Build history of the part. All positions in model axes, mm. A direction names the side the tool comes from. Give positions to 0.01 mm unless a question says otherwise; leave off trailing zeros. Order: outer loops, then holes, each group sorted by start corner. A loop starts at its lowest first (then second) coordinate and runs counter-clockwise, first axis right, second up. Notation, with made-up numbers: (-10, 52.25) - (45, 52.25) arc R22 cw to (45, 58.25) - close; hole circle Ø2 at (86, 55). An arc over 180 degrees is marked (long way). Use a Markdown table: item, result.
from build123d import *

# Parameters (mm, degrees)
F1_DEPTH       = 3
F2_D           = 8
F2_CSINK_D     = 16
F2_CSINK_ANGLE = 90


with BuildPart() as f1:
    # F0 (on Front) → F1 (new body)
    with BuildSketch(Plane.XZ):
        with BuildLine():
            ThreePointArc((-42.428788, 22.197763), (-22.393428, 40.636528), (0.736568, 26.269656))
            Line((0.736568, 26.269656), (7.82161, 7.734496))
            Line((7.82161, 7.734496), (445.831745, 440.866256))
            Line((445.831745, 440.866256), (409.571118, 551.809463))
            ThreePointArc((409.571118, 551.809463), (403.393924, 553.012383), (397.791506, 555.879027))
            Line((397.791506, 555.879027), (-153.711431, 555.879027))
            Line((-153.711431, 555.879027), (-163.711431, 555.879027))
            Line((-163.711431, 555.879027), (-176.433934, 530.299822))
            Line((-176.433934, 530.299822), (-292.672837, 296.595913))
            Line((-292.672837, 296.595913), (-429.805557, 108.635613))
            ThreePointArc((-429.805557, 108.635613), (-433.055197, 105.145969), (-437.038546, 102.524765))
            Line((-437.038546, 102.524765), (-467.979575, 87.098137))
            ThreePointArc((-467.979575, 87.098137), (-479.031049, 77.063624), (-483.216559, 62.73505))
            Line((-483.216559, 62.73505), (-444.218322, 62.364245))
            ThreePointArc((-444.218322, 62.364245), (-439.992581, 60.566627), (-438.27564, 56.307469))
            ThreePointArc((-438.27564, 56.307469), (-440.073258, 52.081729), (-444.332415, 50.364787))
            Line((-444.332415, 50.364787), (-483.330653, 50.735592))
            Line((-483.330653, 50.735592), (-473.742625, 39.200006))
            ThreePointArc((-473.742625, 39.200006), (-462.016917, 29.862605), (-447.542263, 25.968544))
            Line((-447.542263, 25.968544), (-119.640526, 6.942116))
            ThreePointArc((-119.640526, 6.942116), (-119.539343, 30.38703), (-113.982147, 53.164032))
            ThreePointArc((-113.982147, 53.164032), (-112.028876, 55.605369), (-109.00742, 56.409233))
            Line((-109.00742, 56.409233), (-91.138541, 55.372396))
            ThreePointArc((-91.138541, 55.372396), (-94.609764, 47.818656), (-97.278364, 39.945477))
            ThreePointArc((-97.278364, 39.945477), (-100.140537, 22.963258), (-99.30184, 5.761968))
            Line((-99.30184, 5.761968), (-45.922757, 2.664658))
            Line((-45.922757, 2.664658), (-42.428788, 22.197763))
        make_face()
        with BuildLine():
            ThreePointArc((-219.185589, 82.205842), (-234.185589, 97.205842), (-219.185589, 112.205842))
            Line((-219.185589, 112.205842), (-139.185589, 112.205842))
            ThreePointArc((-139.185589, 112.205842), (-124.185589, 97.205842), (-139.185589, 82.205842))
            Line((-139.185589, 82.205842), (-219.185589, 82.205842))
        make_face(mode=Mode.SUBTRACT)
        with BuildLine():
            ThreePointArc((-238.884885, 257.620199), (-269.539195, 249.087128), (-278.072266, 279.741438))
            Line((-278.072266, 279.741438), (-223.998126, 375.532812))
            ThreePointArc((-223.998126, 375.532812), (-193.343817, 384.065883), (-184.810746, 353.411573))
            Line((-184.810746, 353.411573), (-238.884885, 257.620199))
        make_face(mode=Mode.SUBTRACT)
        with BuildLine():
            ThreePointArc((-109.00742, 56.409233), (-99.197738, 50.987949), (-97.278364, 39.945477))
            ThreePointArc((-97.278364, 39.945477), (-94.609764, 47.818656), (-91.138541, 55.372396))
            Line((-91.138541, 55.372396), (-109.00742, 56.409233))
        make_face()
        with BuildLine():
            Line((-153.711431, 555.879027), (397.791506, 555.879027))
            ThreePointArc((397.791506, 555.879027), (388.241023, 574.279027), (397.791506, 592.679027))
            Line((397.791506, 592.679027), (-153.711431, 592.679027))
            ThreePointArc((-153.711431, 592.679027), (-135.311431, 574.279027), (-153.711431, 555.879027))
        make_face()
        with BuildLine():
            Line((-153.711431, 592.679027), (397.791506, 592.679027))
            ThreePointArc((397.791506, 592.679027), (403.393924, 595.545671), (409.571118, 596.748591))
            Line((409.571118, 596.748591), (418.046209, 622.679027))
            Line((418.046209, 622.679027), (406.046209, 622.679027))
            ThreePointArc((406.046209, 622.679027), (403.924889, 623.557707), (403.046209, 625.679027))
            ThreePointArc((403.046209, 625.679027), (403.924889, 627.800347), (406.046209, 628.679027))
            Line((406.046209, 628.679027), (420.007247, 628.679027))
            Line((420.007247, 628.679027), (445.831745, 707.691799))
            Line((445.831745, 707.691799), (7.82161, 1140.823559))
            Line((7.82161, 1140.823559), (0.736568, 1122.288398))
            ThreePointArc((0.736568, 1122.288398), (-22.393428, 1107.921526), (-42.428788, 1126.360291))
            Line((-42.428788, 1126.360291), (-45.922757, 1145.893396))
            Line((-45.922757, 1145.893396), (-447.542263, 1122.58951))
            ThreePointArc((-447.542263, 1122.58951), (-462.016917, 1118.695449), (-473.742625, 1109.358048))
            Line((-473.742625, 1109.358048), (-483.330653, 1097.822462))
            Line((-483.330653, 1097.822462), (-444.332415, 1098.193267))
            ThreePointArc((-444.332415, 1098.193267), (-440.073258, 1096.476326), (-438.27564, 1092.250585))
            ThreePointArc((-438.27564, 1092.250585), (-439.992581, 1087.991428), (-444.218322, 1086.19381))
            Line((-444.218322, 1086.19381), (-483.216559, 1085.823005))
            ThreePointArc((-483.216559, 1085.823005), (-479.031049, 1071.494431), (-467.979575, 1061.459917))
            Line((-467.979575, 1061.459917), (-437.038546, 1046.033289))
            ThreePointArc((-437.038546, 1046.033289), (-433.055197, 1043.412085), (-429.805557, 1039.922441))
            Line((-429.805557, 1039.922441), (-292.672837, 851.962142))
            Line((-292.672837, 851.962142), (-178.632735, 622.679027))
            Line((-178.632735, 622.679027), (-176.433934, 618.258232))
            Line((-176.433934, 618.258232), (-163.711431, 592.679027))
            Line((-163.711431, 592.679027), (-153.711431, 592.679027))
        make_face()
        with BuildLine():
            ThreePointArc((-281.759139, 875.347847), (-276.070425, 895.784053), (-255.634219, 890.095339))
            Line((-255.634219, 890.095339), (-194.186333, 781.241505))
            ThreePointArc((-194.186333, 781.241505), (-199.875047, 760.805298), (-220.311253, 766.494012))
            Line((-220.311253, 766.494012), (-281.759139, 875.347847))
        make_face(mode=Mode.SUBTRACT)
    extrude(amount=-F1_DEPTH)

    # F2 (through all)
    with Locations(Plane.XZ):
        with Locations((386.357424, 494.079027), (-83.001788, 494.079027), (4.204936, 95.571513), (-83.001788, 654.479027), (4.204936, 1052.986541), (386.357424, 654.479027)):
            CounterSinkHole(F2_D / 2, F2_CSINK_D / 2, counter_sink_angle=F2_CSINK_ANGLE)


solid = f1.part
1) Pin check, flat tips, straight feed: P1, Ø1.5, axis at x = 413, y = 2, coming from the -Z side; P2, Ø0.9, axis at x = -157, y = 1.5, coming from the +Z side; P3, Ø1.5, axis at x = -56.5, y = 1.5, coming from the +Z side. Stop position of each tip, or through.
Computed:
| item | result |
|---|---|
| P1 | stops at z = 407.66 |
| P2 | stops at z = 1139.47 |
| P3 | stops at z = 1145.32 |
2) Slice it at B-B (y = 1.6). State how many separate pieces and enclosed holes the cut face has, and give its area (3 significant figures).
Computed:
| item | result |
|---|---|
| separate pieces | 1 |
| enclosed holes | 9 |
| area | 637,000 mm² |
3) Slice it at A-A (z = 822). Write the cut outline in (x, y), and give its area (3 significant figures).
Computed:
| item | result |
|---|---|
| outline | (-277.77, 0) - (-251.64, 0) - (-251.64, 3) - (-277.77, 3) - close; (-217.19, 0) - (330.24, 0) - (330.24, 3) - (-217.19, 3) - close |
| area | 1,720 mm² |
4) Tool access for faces 5 (the flat face through (-362.2, 1.48, 947.26)), 6 (the flat face through (-251.41, 1.48, 326.97)), 7 (the flat face through (223.76, 1.48, 221.27)), 8 (the flat face through (432.74, 1.48, 667.63)): list every direction of +Z, -Z, +X, -X, +Y, -Y with a clear straight run to the whole face (end or side of a thin tool).
Computed:
| item | result |
|---|---|
| face 5 | -X, +Y, -Y |
| face 6 | +Y, -Y |
| face 7 | -Z, +X, +Y, -Y |
| face 8 | +X, +Y, -Y |
5) Two-plate mould, pull along X, no slides. Class faces 1 (the flat face through (427.955, 1.479, 495.561)), 2 (the flat face through (-243.921, 1.479, 1134.405)), 3 (the flat face through (-225.34, 1.48, 836.43)), 4 (the flat face through (-25, 0, 582)): +X half, -X half, draft (parallel to the pull), parting line (faces both ways), or undercut.
Computed:
| item | result |
|---|---|
| face 1 | +X half |
| face 2 | -X half |
| face 3 | undercut |
| face 4 | draft |
6) Slice it at C-C (z = 326.5). Write the cut outline in (x, y).
Computed:
| item | result |
|---|---|
| outline | (-277.8, 0) - (-251.68, 0) - (-251.68, 3) - (-277.8, 3) - close; (-200, 0) - (330.18, 0) - (330.18, 3) - (-200, 3) - close |
7) Wall check: line 1 (Z direction, x = -78.5, y = 2.2); line 2 (Z direction, x = -294, y = 1.45); line 3 (Z direction, x = 402, y = 1.5). Give the ranges that are in metal, low to high. Write a range as from..to.
Computed:
| item | result |
|---|---|
| line 1 | z = 4.55..490.42, 497.74..650.82, 658.14..1144 |
| line 2 | z = 17.06..294.78, 853.78..1131.5 |
| line 3 | z = 397.52..553.55, 595.01..751.04 |
8) Slice it at D-D (x = 152). Write the cut outline in (y, z), and give its area (3 significant figures).
Computed:
| item | result |
|---|---|
| outline | (0, 150.31) - (3, 150.31) - (3, 998.25) - (0, 998.25) - close |
| area | 2,540 mm² |
